Print and shaded views of the part. All mm, measured from the part's lowest x, y and z. A direction names the side the tool comes from. Coordinates: 2 decimals unless noted, no trailing zeros. Order: outer loops, then holes, each group sorted by start corner. A loop starts at its lowest first (then second) coordinate and runs counter-clockwise, first axis right, second up.
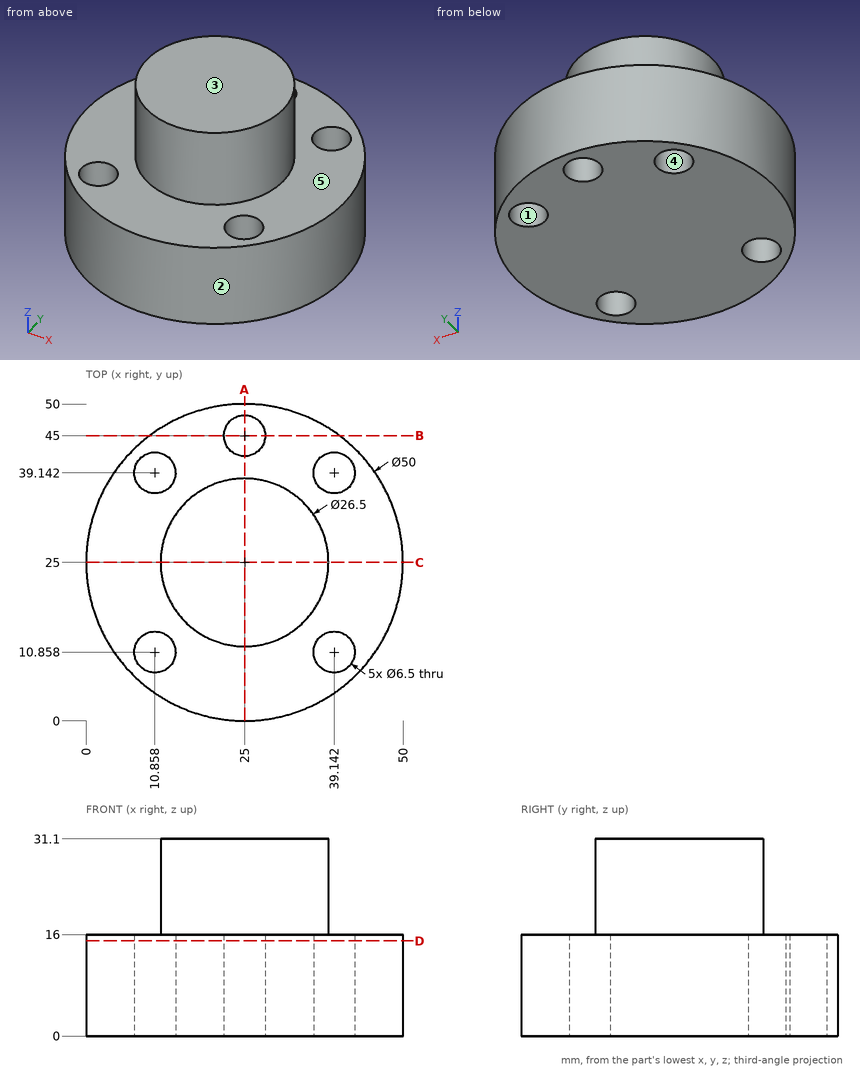
Q1. Probe line 1 (X direction, y = 38.5, z = 13); line 2 (Y direction, x = 25, z = 5); line 3 (Y direction, x = 9, z = 9.5) (1 decimal). List the from-to ranges inside material, lowest first.
Established:
line 1: x = 3.96 to 7.67, 14.04 to 35.96, 42.33 to 46.04
line 2: y = 0 to 41.75, 48.25 to 50
line 3: y = 5.8 to 8.2, 13.5 to 36.5, 41.8 to 44.2
Q2. Which spindle directions (+Z, -Z, +X, -X, +Y, -Y) get a long thin tool onto all of the face, cutting with end or side? Do the marked faces 4 and 5. Say none if no direction does.
Established:
face 4: +Z, -Z
face 5: +Z
Q3. Mould opens along X. For the marked faces 1, 2 and 3 say: pulls with the +X half, pulls with the -X half, needs draft (parallel to the pull), parting line crosses it, or undercut.
Established:
face 1: undercut
face 2: parting line crosses it
face 3: needs draft
Q4. Cut at A-A, the plane x = 25. List the corners of the cut face in (y, z), plus the area to 3 significant figures.
Established:
outline: (0, 0) - (41.75, 0) - (41.75, 16) - (38.25, 16) - (38.25, 31.1) - (11.75, 31.1) - (11.75, 16) - (0, 16) - close; (48.25, 0) - (50, 0) - (50, 16) - (48.25, 16) - close
area: 1,100 mm2
Q5. Cut at C-C, the plane y = 25. List the corners of the cut face in (x, z).
Established:
outline: (0, 0) - (50, 0) - (50, 16) - (38.25, 16) - (38.25, 31.1) - (11.75, 31.1) - (11.75, 16) - (0, 16) - close
Q6. Cut at B-B, the plane y = 45. List the corners of the cut face in (x, z).
Established:
outline: (10, 0) - (21.75, 0) - (21.75, 16) - (10, 16) - close; (28.25, 0) - (40, 0) - (40, 16) - (28.25, 16) - close
Q7. Drop flat-ended pins along their axis: P1, Ø1, axis at x = 21.5, z = 21.5, coming from the -Y side; P2, Ø5, axis at x = 27, z = 27, coming from the -Y side; P3, Ø5, axis at x = 10.86, y = 39.14, coming from the -Z side; P4, Ø1, axis at y = 18, z = 25.5, coming from the -X side. Give the stop position or say it passes through.
Established:
P1: stops at y = 12.09
P2: stops at y = 11.75
P3: passes through
P4: stops at x = 13.45
Q8. Cut at D-D, the plane z = 15. List the corners of the cut face in (x, y).
Established:
outline: circle Ø50 at (25, 25); hole circle Ø6.5 at (10.86, 10.86); hole circle Ø6.5 at (10.86, 39.14); hole circle Ø6.5 at (25, 45); hole circle Ø6.5 at (39.14, 10.86); hole circle Ø6.5 at (39.14, 39.14)
